Print and shaded views of the part. All mm, measured from the part's lowest x, y and z. A direction names the side the tool comes from. Round coordinates to 2 decimals unless told otherwise and drop trailing zeros. Write each loop counter-clockwise with the first axis right and the second up, starting at its lowest first coordinate (ties: lowest second). Pieces come first, ordered by that corner, then holes.
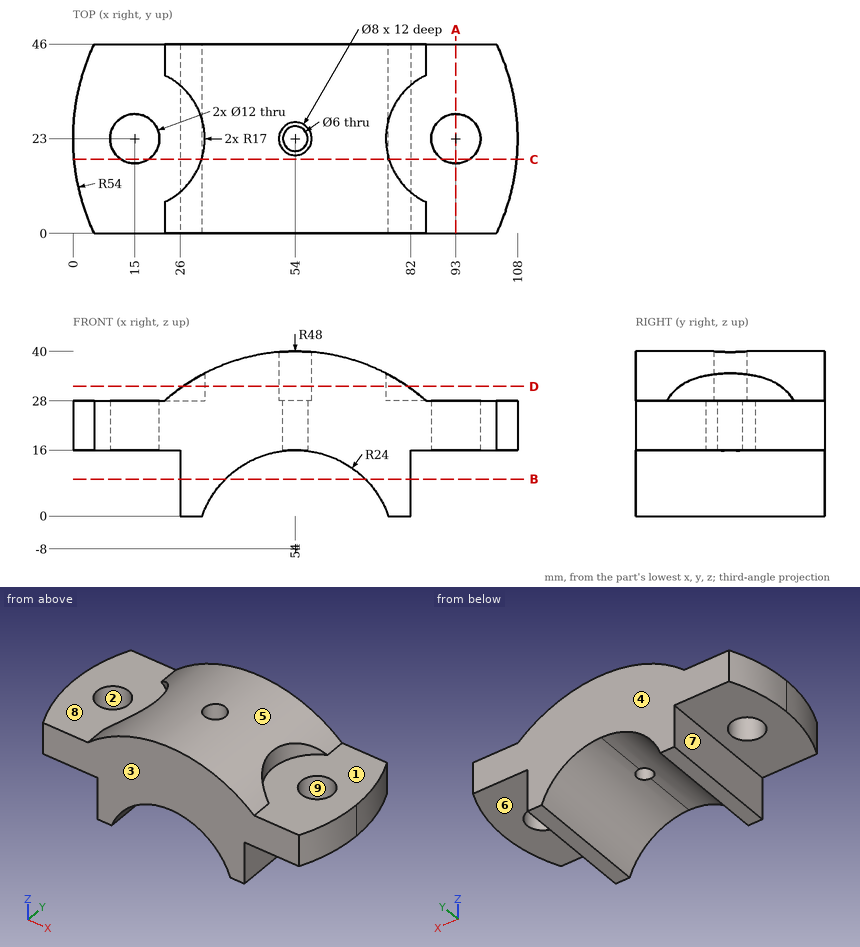
1) Slice it at B-B (z = 9). Write the cut outline in (x, y).
Results:
outline: (26, 0) - (37.06, 0) - (37.06, 46) - (26, 46) - close; (70.94, 0) - (82, 0) - (82, 46) - (70.94, 46) - close
2) Wall check: L1, parallel to Y at x = 54, z = 35.5; L2, parallel to Y at x = 54, z = 22.25; L3, parallel to Z at x = 96, y = 14.5. Give the ranges that are in metal, low to high.
Results:
L1: y = 0 to 19, 27 to 46
L2: y = 0 to 20, 26 to 46
L3: z = 16 to 28
3) Pin check, flat tips, straight feed: pin 1 Ø5 at (y, z) = (33.5, 18.5) entering from -X; pin 2 Ø4 at (x, y) = (73.5, 19.5) entering from -Z; pin 3 Ø5 at (x, y) = (68, 10) entering from -Z. Stop position of each tip, or through.
Results:
pin 1: stops at x = 0.6
pin 2: stops at z = 2.67
pin 3: stops at z = 9.43
4) Slice it at D-D (z = 31.5). Write the cut outline in (x, y), plus the area to 3 significant figures.
Results:
outline: (26.73, 0) - (81.27, 0) - (81.27, 10.69) arc R17 cw to (81.27, 35.31) - (81.27, 46) - (26.73, 46) - (26.73, 35.31) arc R17 cw to (26.73, 10.69) - close; hole circle Ø8 at (54, 23)
area: 2,280 mm2
5) Which spindle directions (+Z, -Z, +X, -X, +Y, -Y) get a long thin tool onto all of the face, cutting with end or side? Do the marked faces 5, 6, 7, 8 and 9. Say none if no direction does.
Results:
face 5: +Z, +Y, -Y
face 6: -Z, +X, +Y, -Y
face 7: -Z, -X, +Y, -Y
face 8: +Z, -X
face 9: +Z, -Z
6) Mould opens along Y. For the marked faces 1, 2, 3 and 4 say: released by +Y, released by -Y, zero draft, split by the parting line, or undercut.
Results:
face 1: undercut
face 2: undercut
face 3: released by -Y
face 4: released by +Y
7) Slice it at C-C (y = 18). Write the cut outline in (x, z).
Results:
outline: (0.23, 16) - (11.68, 16) - (11.68, 28) - (0.23, 28) - close; (18.32, 16) - (26, 16) - (26, 0) - (31.37, 0) arc R24 cw to (76.63, 0) - (82, 0) - (82, 16) - (89.68, 16) - (89.68, 28) - (76.75, 28) - (76.75, 34.27) arc R48 ccw to (31.25, 34.27) - (31.25, 28) - (18.32, 28) - close; (96.32, 16) - (107.77, 16) - (107.77, 28) - (96.32, 28) - close
8) Slice it at A-A (x = 93). Write the cut outline in (y, z), plus the area to 3 significant figures.
Results:
outline: (0, 16) - (17, 16) - (17, 28) - (0, 28) - close; (29, 16) - (46, 16) - (46, 28) - (29, 28) - close
area: 408 mm2
